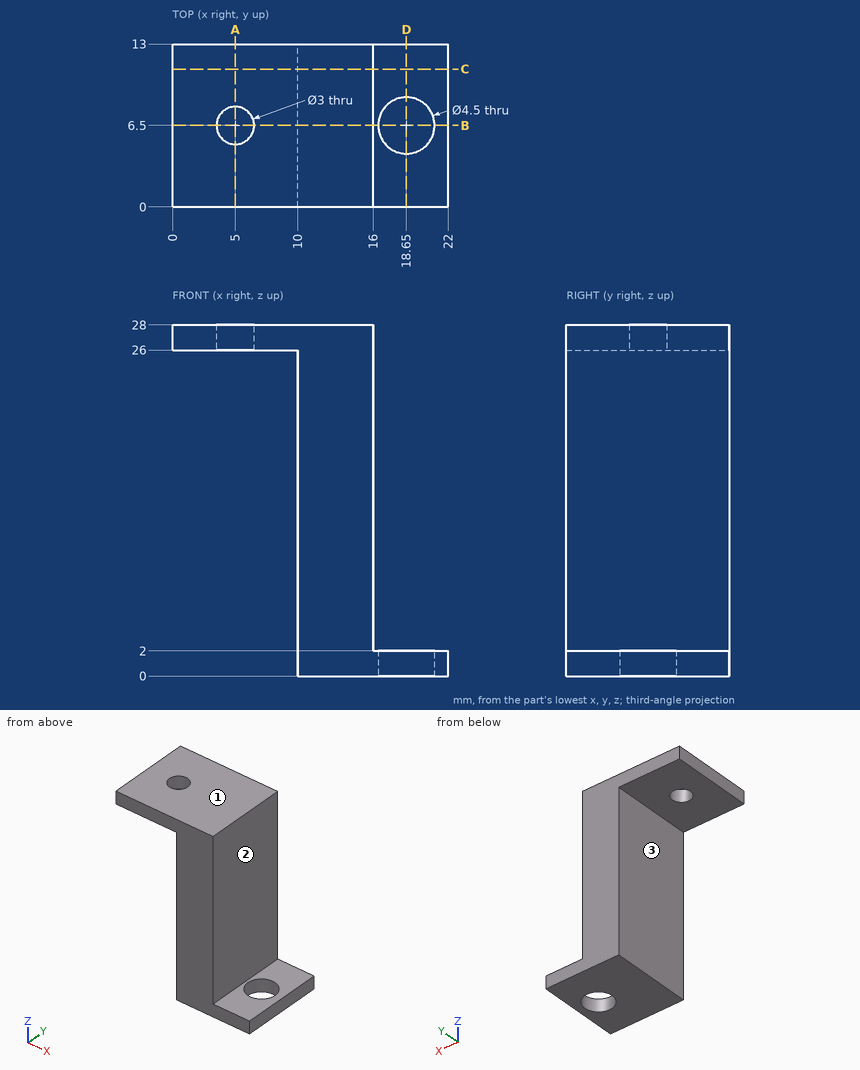
The drawing under review shows one solid part. Ordinate dimensions are in mm from its lowest x, y, z. A direction names the side the tool comes from. Give positions to 0.01 mm unless a question says otherwise; leave off trailing zeros. Write each loop counter-clockwise with the first axis right and the second up, starting at its lowest first coordinate (ties: lowest second). Pieces come first, ordered by that corner, then holes. Notation, with made-up numbers: (57, 44) - (70, 44) arc R15 ccw to (70, 60) - close; hole circle Ø11 at (43.25, -36.5). An arc over 180 degrees is marked (long way). Answer in a Markdown table with one row per item. Add a question column.
1. We need section A-A on x = 5. Write out the cut boundary in (y, z), then the cut area to 3 significant figures.
2. Insertion check: P1, Ø2.5, axis at x = 5, y = 6.5, coming from the +Z side; P2, Ø6, axis at y = 7.5, z = 9.5, coming from the -X side; P3, Ø5, axis at x = 4.5, y = 4.5, coming from the -Z side; P4, Ø2, axis at y = 5.5, z = 11.5, coming from the +X side. Each pin has a flat end and moves straight along its axis. Give the tip position at first contact, or say it passes through.
3. We need section C-C on y = 11. Write out the cut boundary in (x, z).
4. We need section B-B on y = 6.5. Write out the cut boundary in (x, z).
5. Tool access review of the marked faces 1, 2 and 3: name each direction out of +Z, -Z, +X, -X, +Y, -Y from which nothing blocks a thin tool from reaching the whole face with its end or side.
6. We need section D-D on x = 18.65. Write out the cut boundary in (y, z).
7. Wall thickness on line 1 along Y through (x, z) = (18.65, 0.55); line 2 along Y through (x, z) = (5, 26.9); line 3 along X through (y, z) = (10.5, 10.75): over which ranges is each line inside the solid? List them lowest first. Write a range as [from, to].
Ans:
| question | item | result |
|---|---|---|
| 1 | outline | (0, 26) - (5, 26) - (5, 28) - (0, 28) - close; (8, 26) - (13, 26) - (13, 28) - (8, 28) - close |
| 1 | area | 20.0 mm^2 |
| 2 | P1 | passes through |
| 2 | P2 | stops at x = 10 |
| 2 | P3 | stops at z = 26 |
| 2 | P4 | stops at x = 16 |
| 3 | outline | (0, 26) - (10, 26) - (10, 0) - (22, 0) - (22, 2) - (16, 2) - (16, 28) - (0, 28) - close |
| 4 | outline | (0, 26) - (3.5, 26) - (3.5, 28) - (0, 28) - close; (6.5, 26) - (10, 26) - (10, 0) - (16.4, 0) - (16.4, 2) - (16, 2) - (16, 28) - (6.5, 28) - close; (20.9, 0) - (22, 0) - (22, 2) - (20.9, 2) - close |
| 5 | face 1 | +Z, +X, -X, +Y, -Y |
| 5 | face 2 | +Z, +X, +Y, -Y |
| 5 | face 3 | -Z, -X, +Y, -Y |
| 6 | outline | (0, 0) - (4.25, 0) - (4.25, 2) - (0, 2) - close; (8.75, 0) - (13, 0) - (13, 2) - (8.75, 2) - close |
| 7 | line 1 | y = [0, 4.25], [8.75, 13] |
| 7 | line 2 | y = [0, 5], [8, 13] |
| 7 | line 3 | x = [10, 16] |
